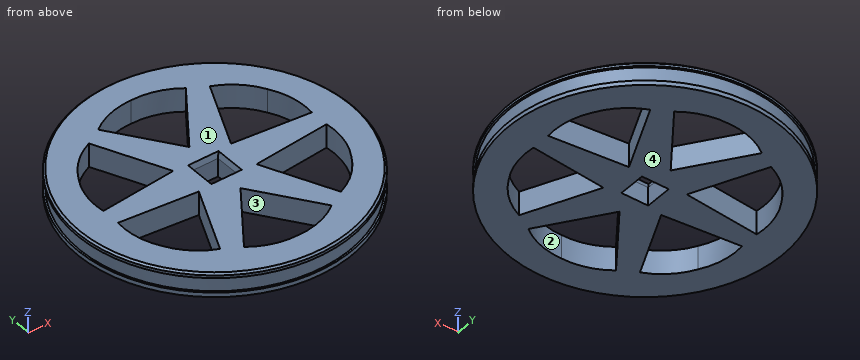
```python
from build123d import *

# Parameters (mm, degrees)
SKETCH1_R           = 37.5
SKETCH1_W           = 7.35
SKETCH1_H           = 7.35
BOSS_EXTRUDE1_DEPTH = 3.25
CUT_EXTRUDE1_DEPTH  = 4
CIRPATTERN1_COUNT   = 6
SKETCH3_R           = 37.5
SKETCH3_R_2         = 37
CUT_EXTRUDE2_DEPTH  = 2
CHAMFER1_SIZE       = 0.5
CHAMFER1_SIZE2      = 1.5
CHAMFER2_SIZE       = 0.5


with BuildPart() as part:
    # Sketch1 → Boss-Extrude1 (new, symmetric)
    with BuildSketch(Plane.XY):
        with Locations(Location((0, 0, 0), (0, 0, 180))):
            Circle(SKETCH1_R)
        Rectangle(SKETCH1_W, SKETCH1_H, mode=Mode.SUBTRACT)
    extrude(amount=BOSS_EXTRUDE1_DEPTH, both=True)

    # Sketch2 → Cut-Extrude1 (cut, symmetric)
    with BuildSketch(Plane.XY):
        with BuildLine():
            Line((0, 9.158641407), (-12.037071564, 26.115211784))
            ThreePointArc((-12.037071564, 26.115211784), (-6.351662121, 29.087034336), (0, 29.988143709))
            ThreePointArc((0, 29.988143709), (6.351662121, 29.087034336), (12.037071564, 26.115211784))
            Line((12.037071564, 26.115211784), (0, 9.158641407))
        make_face()
    cut_extrude1 = extrude(amount=CUT_EXTRUDE1_DEPTH, both=True, mode=Mode.SUBTRACT)

    # CirPattern1: Cut-Extrude1 ×6 about axis
    cirpattern1_axis = Axis((0, 0, 0), (0, 0, 1))
    for i in range(1, CIRPATTERN1_COUNT):
        add(cut_extrude1.rotate(cirpattern1_axis, i * 360 / CIRPATTERN1_COUNT), mode=Mode.SUBTRACT)

    # Sketch3 → Cut-Extrude2 (cut, symmetric)
    with BuildSketch(Plane.XY):
        with Locations(Location((0, 0, 0), (0, 0, 180))):
            Circle(SKETCH3_R)
        Circle(SKETCH3_R_2, mode=Mode.SUBTRACT)
    extrude(amount=CUT_EXTRUDE2_DEPTH, both=True, mode=Mode.SUBTRACT)

    # Chamfer1
    chamfer1_edges = [part.edges().sort_by_distance(p)[0] for p in [
        (3.675, 0, 3.25),
        (0, 3.675, 3.25),
        (-3.675, 0, 3.25),
        (0, -3.675, 3.25),
    ]]
    chamfer1_side = [part.faces().sort_by_distance(p)[0] for p in [
        (36.439339828, 0, 3.25),
    ]]
    chamfer(chamfer1_edges, length=CHAMFER1_SIZE, length2=CHAMFER1_SIZE2, reference=chamfer1_side[0])

    # Chamfer2
    chamfer2_edges = [part.edges().sort_by_distance(p)[0] for p in [
        (37.5, 0, 3.25),
    ]]
    chamfer(chamfer2_edges, length=CHAMFER2_SIZE)


solid = part.part
```
Build history of the part. All positions in model axes, mm. Face numbers are marked on the shaded views. A direction names the side the tool comes from. Round coordinates to 2 decimals unless told otherwise and drop trailing zeros. Order: outer loops, then holes, each group sorted by start corner. A loop starts at its lowest first (then second) coordinate and runs counter-clockwise, first axis right, second up. Notation, with made-up numbers: (5, 23) -> (28, 23) arc R23 ccw to (28, 46) -> close; hole circle Ø9 at (-31.75, 50). An arc over 180 degrees is marked (long way). Answer in a Markdown table with one row per item.
1) Band-saw the part on A-A on y = 0. Give the cut face in (x, z) (3 decimals).
Values:
| item | result |
|---|---|
| outline | (-37.5, -3.25) -> (-3.675, -3.25) -> (-3.675, 1.75) -> (-4.175, 3.25) -> (-37, 3.25) -> (-37.5, 2.75) -> (-37.5, 2) -> (-37, 2) -> (-37, -2) -> (-37.5, -2) -> close; (3.675, -3.25) -> (37.5, -3.25) -> (37.5, -2) -> (37, -2) -> (37, 2) -> (37.5, 2) -> (37.5, 2.75) -> (37, 3.25) -> (4.175, 3.25) -> (3.675, 1.75) -> close |
2) Mould opens along Y. For the marked faces 1 and 2 say: released by +Y, released by -Y, zero draft, split by the parting line, or undercut.
Values:
| item | result |
|---|---|
| face 1 | zero draft |
| face 2 | undercut |
3) Pin check, flat tips, straight feed: P1, Ø1.5, axis at y = -24, z = -1.5, coming from the +X side; P2, Ø22.5, axis at x = -17.5, y = -5.5, coming from the -Z side; P3, Ø2.5, axis at x = -1.5, z = -0.5, coming from the -Y side; P4, Ø1.5, axis at y = -1.5, z = -0.5, coming from the -X side. Stop position of each tip, or through.
Values:
| item | result |
|---|---|
| P1 | x = 29.27 |
| P2 | z = -3.25 |
| P3 | y = -37 |
| P4 | x = -36.99 |
4) Which spindle directions (+Z, -Z, +X, -X, +Y, -Y) get a long thin tool onto all of the face, cutting with end or side? Do the marked faces 3 and 4. Say none if no direction does.
Values:
| item | result |
|---|---|
| face 3 | +Z, -Z |
| face 4 | -Z, +X, -X, +Y, -Y |
5) Band-saw the part on B-B on x = -13. Give the number of separate pieces and of enclosed holes in the cut face, and give its area (3 significant figures).
Values:
| item | result |
|---|---|
| separate pieces | 3 |
| enclosed holes | 0 |
| area | 303 mm2 |
6) Wall check: L1, parallel to X at y = 22, z = 2.25; L2, parallel to Y at x = -19, z = 2.5; L3, parallel to X at y = -22, z = -1.25. Give the ranges that are in metal, low to high.
Values:
| item | result |
|---|---|
| L1 | -30.37 to -19.44, -15.92 to -9.12, 9.12 to 15.92, 19.44 to 30.37 |
| L2 | -32.33 to -22.27, -3.54 to 3.54, 22.27 to 32.33 |
| L3 | -29.75 to -19.44, -15.92 to -9.12, 9.12 to 15.92, 19.44 to 29.75 |
